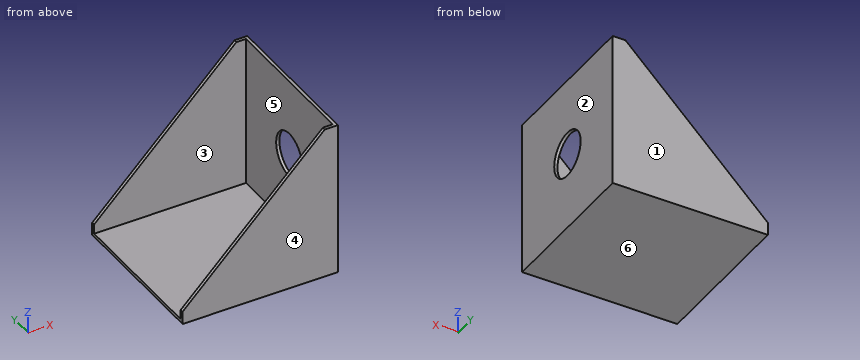
```python
from build123d import *

# Parameters (mm, degrees)
F1_DEPTH = 76.2
F2_T     = -1.5875
F3_R     = 11.1125
F4_DEPTH = 1.5885


with BuildPart() as f1:
    # F0 (on Front) → F1 (new body)
    with BuildSketch(Plane.XZ):
        Polygon((-76.2, 0), (0, 0), (0, 76.2), (-6.35, 76.2), (-76.2, 6.35), align=None)
    extrude(amount=F1_DEPTH)

    # F2
    f2_openings = [f1.faces().sort_by_distance(p)[0] for p in [
        (-41.275, -38.1, 41.275),
        (-76.2, -38.1, 3.175),
        (-3.175, -38.1, 76.2),
    ]]
    offset(amount=F2_T, openings=f2_openings)

    # F3 (on face) → F4 (cut, through all)
    with BuildSketch(Plane(origin=(-1.5875, 0, 0), x_dir=(0, -1, 0), z_dir=(-1, 0, 0))):
        with Locations((38.1, 38.1)):
            Circle(F3_R)
    extrude(amount=-F4_DEPTH, mode=Mode.SUBTRACT)


solid = f1.part
```
The model under review builds one solid part; all positions refer to its coordinate system, in mm. Face numbers are marked on the shaded views. A direction names the side the tool comes from. Round coordinates to 2 decimals unless told otherwise and drop trailing zeros. Loops run counter-clockwise (first coordinate to the right, second up) from the corner with the lowest first, then second, coordinate; pieces in that order, holes last. Notation, with made-up numbers: (65, -21) -> (80, -21) arc R23 cw to (80, 7) -> close; hole circle Ø9 at (62.5, -31.5). An arc over 180 degrees is marked (long way). Answer in a Markdown table with one row per item.
1) For pin 1 Ø12 at (x, y) = (-11, -67) entering from +Z; pin 2 Ø12 at (y, z) = (-27.5, 28) entering from -X, all flat-tipped, find the tip position at first contact; note any pin that passes through.
Taken from the geometry:
| item | result |
|---|---|
| pin 1 | stops at z = 1.59 |
| pin 2 | stops at x = -1.59 |
2) Consider section A-A, the plane y = -38.1. Write out the cut boundary in (x, z), plus the area to 3 significant figures.
Taken from the geometry:
| item | result |
|---|---|
| outline | (-76.2, 0) -> (0, 0) -> (0, 26.99) -> (-1.59, 26.99) -> (-1.59, 1.59) -> (-76.2, 1.59) -> close; (-1.59, 49.21) -> (0, 49.21) -> (0, 76.2) -> (-1.59, 76.2) -> close |
| area | 204 mm² |
3) Tool access review of the marked faces 5 and 6: name each direction out of +Z, -Z, +X, -X, +Y, -Y from which nothing blocks a thin tool from reaching the whole face with its end or side.
Taken from the geometry:
| item | result |
|---|---|
| face 5 | +Z, -X |
| face 6 | -Z, +X, -X, +Y, -Y |
4) Consider section B-B, the plane x = -52. Write out the cut boundary in (y, z).
Taken from the geometry:
| item | result |
|---|---|
| outline | (-76.2, 0) -> (0, 0) -> (0, 30.55) -> (-1.59, 30.55) -> (-1.59, 1.59) -> (-74.61, 1.59) -> (-74.61, 30.55) -> (-76.2, 30.55) -> close |
5) Draft analysis for pull direction Y (two halves, no side actions). For the marked faces 1, 2, 3 and 4, state which applies: pulls with the +Y half, pulls with the -Y half, needs draft (parallel to the pull), parting line crosses it, or undercut.
Taken from the geometry:
| item | result |
|---|---|
| face 1 | pulls with the +Y half |
| face 2 | needs draft |
| face 3 | undercut |
| face 4 | pulls with the -Y half |
6) Consider section D-D, the plane z = 53.5. Write out the cut boundary in (x, y), plus the area to 3 significant figures.
Taken from the geometry:
| item | result |
|---|---|
| outline | (-29.05, -76.2) -> (0, -76.2) -> (0, 0) -> (-29.05, 0) -> (-29.05, -1.59) -> (-1.59, -1.59) -> (-1.59, -74.61) -> (-29.05, -74.61) -> close |
| area | 208 mm² |
7) Consider section C-C, the plane z = 38.1. Write out the cut boundary in (x, y), plus the area to 3 significant figures.
Taken from the geometry:
| item | result |
|---|---|
| outline | (-44.45, -76.2) -> (0, -76.2) -> (0, -49.21) -> (-1.59, -49.21) -> (-1.59, -74.61) -> (-44.45, -74.61) -> close; (-44.45, -1.59) -> (-1.59, -1.59) -> (-1.59, -26.99) -> (0, -26.99) -> (0, 0) -> (-44.45, 0) -> close |
| area | 222 mm² |
8) Wall thickness on line 1 along Y through (x, z) = (-26.5, 24); line 2 along Z through (x, y) = (-0.9, -38.1); line 3 along Y through (x, z) = (-1, 38): over which ranges is each line inside the solid? List them lowest first.
Taken from the geometry:
| item | result |
|---|---|
| line 1 | y = -76.2 to -74.61, -1.59 to 0 |
| line 2 | z = 0 to 26.99, 49.21 to 76.2 |
| line 3 | y = -76.2 to -49.21, -26.99 to 0 |
